from build123d import *

# Parameters (mm, degrees)
SKETCH2_R           = 16.5
SKETCH2_R_2         = 15
BOSS_EXTRUDE1_DEPTH = 300
CUT_EXTRUDE1_DEPTH  = 28
SKETCH4_R           = 4
CUT_EXTRUDE2_DEPTH  = 30


with BuildPart() as part:
    # Sketch2 → Boss-Extrude1 (new body)
    with BuildSketch(Plane(origin=(0, 0, 0), x_dir=(1, 0, 0), z_dir=(0, 1, 0))):
        with Locations(Location((0, 0, 0), (0, 0, 270))):
            Circle(SKETCH2_R)
        with Locations(Location((0, 0, 0), (0, 0, 270))):
            Circle(SKETCH2_R_2, mode=Mode.SUBTRACT)
    extrude(amount=BOSS_EXTRUDE1_DEPTH)

    # Sketch3 → Cut-Extrude1 (cut)
    with BuildSketch(Plane(origin=(0, 0, 0), x_dir=(0, 0, -1), z_dir=(1, 0, 0))):
        Polygon((21.27756657, 178), (21.27756657, 122), (-16.5, 122), (-16.5, 150), (-16.5, 178), (-14, 178), align=None)
    extrude(amount=CUT_EXTRUDE1_DEPTH, mode=Mode.SUBTRACT)

    # Sketch4 → Cut-Extrude2 (cut)
    with BuildSketch(Plane(origin=(0, 0, 0), x_dir=(0, 0, -1), z_dir=(1, 0, 0))):
        with Locations((0, 150)):
            Circle(SKETCH4_R)
    extrude(amount=-CUT_EXTRUDE2_DEPTH, mode=Mode.SUBTRACT)


solid = part.part
Build history of the part. All positions in model axes, mm. A direction names the side the tool comes from. Give positions to 0.01 mm unless a question says otherwise; leave off trailing zeros. Write each loop counter-clockwise with the first axis right and the second up, starting at its lowest first coordinate (ties: lowest second). Pieces come first, ordered by that corner, then holes. Notation, with made-up numbers: (-40, 81.25) - (-19, 81.25) arc R17 ccw to (-19, 100.25) - close; hole circle Ø9 at (-13, -14.5). An arc over 180 degrees is marked (long way). Use one line per item in the form item = value. Start each with the question number.
1. Drop flat-ended pins along their axis: pin 1 Ø0.5 at (y, z) = (151.5, 15.5) entering from +X; pin 2 Ø7 at (y, z) = (150, 0) entering from +X; pin 3 Ø3 at (y, z) = (168.5, 1.5) entering from +X; pin 4 Ø2 at (x, y) = (-11.5, 236) entering from -Z. Give the stop position or say it passes through.
2. Probe line 1 (Y direction, x = -16, z = 0); line 2 (Y direction, x = 15, z = -3.5); line 3 (Z direction, x = 0, y = 113). List the from-to ranges inside material, lowest first. Write a range as [from, to].
3. Band-saw the part on A-A on z = 0. Write the cut outline in (x, y), plus the area to 3 significant figures.
4. 3-axis set-ups, long thin cutter, end or side, ignore diameter. For faces 4 (the face through (-13.31, 147.9, 6.92)), 5 (the face through (15, 178, -3)): which of +Z, -Z, +X, -X, +Y, -Y reach the whole face in a straight line?
5. Two-plate mould, pull along Y, no slides. Class faces 1 (the face through (-14.64, 147.9, 7.61)), 2 (the face through (-15, 0, 4)), 3 (the face through (15, 122, -3)): released by +Y, released by -Y, zero draft, split by the parting line, or undercut.
6. Band-saw the part on D-D on y = 195. Write the cut outline in (x, z), plus the area to 3 significant figures.
7. Band-saw the part on B-B on x = -8. Write the cut outline in (y, z), plus the area to 3 significant figures.
8. Band-saw the part on C-C on y = 150. Write the cut outline in (x, z).
Conclusion:
q1.pin_1 = 0
q1.pin_2 = through
q1.pin_3 = -14.7
q1.pin_4 = -12.73
q2.line_1 = [0, 146], [154, 300]
q2.line_2 = [0, 122], [178, 300]
q2.line_3 = [-16.5, -15], [15, 16.5]
q3.outline = (-16.5, 0) - (-15, 0) - (-15, 146) - (-16.5, 146) - close; (-16.5, 154) - (-15, 154) - (-15, 300) - (-16.5, 300) - close; (15, 0) - (16.5, 0) - (16.5, 122) - (15, 122) - close; (15, 178) - (16.5, 178) - (16.5, 300) - (15, 300) - close
q3.area = 804 mm²
q4.face_4 = +Y, -Y
q4.face_5 = +Z, -Z, +X
q5.face_1 = zero draft
q5.face_2 = released by -Y
q5.face_3 = undercut
q6.outline = circle Ø33 at (0, 0); hole circle Ø30 at (0, 0)
q6.area = 148 mm²
q7.outline = (0, -14.43) - (300, -14.43) - (300, -12.69) - (0, -12.69) - close; (0, 12.69) - (300, 12.69) - (300, 14.43) - (0, 14.43) - close
q7.area = 1,050 mm²
q8.outline = (-16.01, -4) arc R16.5 ccw to (0, -16.5) - (0, -15) arc R15 cw to (-14.46, -4) - close; (-16.01, 4) - (-14.46, 4) arc R15 cw to (0, 15) - (0, 16.5) arc R16.5 ccw to start
